```python
from build123d import *
from OCP.BRepFilletAPI import BRepFilletAPI_MakeChamfer

# Parameters (mm, degrees)
EXTRUDE_1_DEPTH     = 25
SKETCH_2_W          = 25
SKETCH_2_H          = 113.275398007
CUT_EXTRUDE_1_DEPTH = 10
EXTRUDE_1_2_DEPTH   = 25
FILLET_1_R          = 50
FILLET_2_R          = 5
CHAMFER_1_SIZE      = 3
CHAMFER_1_SIZE2     = 5.018091596
CHAMFER_1_SIZE2_2   = 4.946391741
EXTRUDE_2_DEPTH     = 25
FILLET_3_R          = 10
CHAMFER_2_SIZE      = 5


with BuildPart() as part:
    # 草图1 → Extrude 1 (new body)
    with BuildSketch(Plane.XY):
        Polygon((-40.289701428, 251), (6, 121.036629463), (6, -6), (-106, -6), (-106, 121.057565217), (-58.723691593, 251), align=None)
        Polygon((-44.521873006, 245), (0, 120), (0, 0), (-100, 0), (-100, 120), (-54.521873006, 245), align=None, mode=Mode.SUBTRACT)
    extrude(amount=EXTRUDE_1_DEPTH)

    # 草图2 → 切除-拉伸1 (cut)
    with BuildSketch(Plane(origin=(-132.504349732, 48.208397155, 0), x_dir=(0, 0, 1), z_dir=(-0.9397364726914574, 0.34189963716479416, 0))):
        with Locations((12.5, 134.158546794)):
            Rectangle(SKETCH_2_W, SKETCH_2_H)
    extrude(amount=-CUT_EXTRUDE_1_DEPTH, mode=Mode.SUBTRACT)

    # 草图4 → Extrude 1 2 (add)
    with BuildSketch(Plane.XY.offset(25)):
        Polygon((-58.077318346, 235.22759518), (-41.041186875, 235.22759518), (-39.260311955, 230.22759518), (-59.896443426, 230.22759518), align=None)
    extrude(amount=-EXTRUDE_1_2_DEPTH)

    # 圆角1
    fillet_1_edges = [part.edges().sort_by_distance(p)[0] for p in [
        (6, 121.036629463, 12.5),
    ]]
    fillet(fillet_1_edges, radius=FILLET_1_R)

    # 圆角2
    fillet_2_edges = [part.edges().sort_by_distance(p)[0] for p in [
        (-58.723691593, 251, 12.5),
        (-40.289701428, 251, 12.5),
    ]]
    fillet(fillet_2_edges, radius=FILLET_2_R)

    # 倒角1: one chamfer whose edges measure the first distance from different faces: ONE call of the kernel's chamfer builder (chamfer() names one face for all edges)
    chamfer_1_edges_1 = [part.edges().sort_by_distance(p)[0] for p in [
        (-59.896443426, 230.22759518, 12.5),
    ]]
    chamfer_1_side_1 = [part.faces().sort_by_distance(p)[0] for p in [
        (-49.57837769, 230.22759518, 12.5),
    ]]
    chamfer_1_edges_2 = [part.edges().sort_by_distance(p)[0] for p in [
        (-39.260311955, 230.22759518, 12.5),
    ]]
    chamfer_1_side_2 = [part.faces().sort_by_distance(p)[0] for p in [
        (-19.630155978, 175.11379759, 12.5),
    ]]
    chamfer_1 = BRepFilletAPI_MakeChamfer(part.part.solid().wrapped)
    for e in chamfer_1_edges_1:
        chamfer_1.Add(CHAMFER_1_SIZE, CHAMFER_1_SIZE2, e.wrapped, chamfer_1_side_1[0].wrapped)  # the first distance lies on this face
    for e in chamfer_1_edges_2:
        chamfer_1.Add(CHAMFER_1_SIZE, CHAMFER_1_SIZE2_2, e.wrapped, chamfer_1_side_2[0].wrapped)  # the first distance lies on this face
    add(Compound.cast(chamfer_1.Shape()), mode=Mode.REPLACE)

    # 草图5 → 凸台-拉伸2 (add)
    with BuildSketch(Plane.XY.offset(25)):
        Polygon((-106, 121.057565217), (-94.163375331, 130.992259513), (-90.60862045, 126.756970729), (-100, 118.874615121), align=None)
    extrude(amount=-EXTRUDE_2_DEPTH)

    # 圆角3
    fillet_3_edges = [part.edges().sort_by_distance(p)[0] for p in [
        (-106, 121.057565217, 12.5),
    ]]
    fillet(fillet_3_edges, radius=FILLET_3_R)

    # 倒角2
    chamfer_2_edges = [part.edges().sort_by_distance(p)[0] for p in [
        (0, 0, 12.5),
        (-100, 0, 12.5),
    ]]
    chamfer(chamfer_2_edges, length=CHAMFER_2_SIZE)


solid = part.part
```
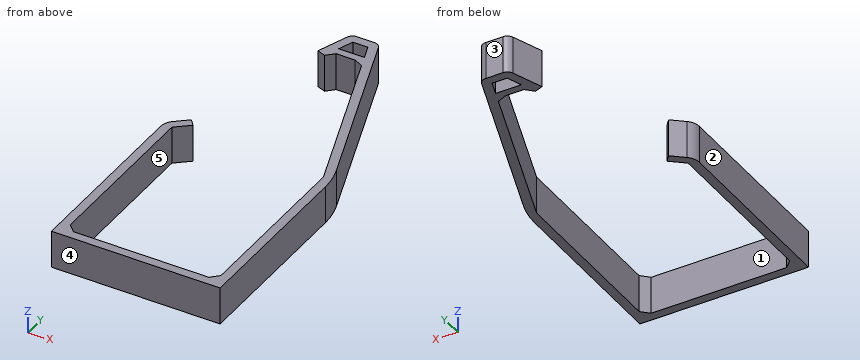
Model file for the job. Use its own axes, mm. Face numbers are marked on the shaded views. A direction names the side the tool comes from. Coordinates: 2 decimals unless noted, no trailing zeros. Write each loop counter-clockwise with the first axis right and the second up, starting at its lowest first coordinate (ties: lowest second). Pieces come first, ordered by that corner, then holes. Notation, with made-up numbers: (81, -38.75) - (109, -38.75) arc R14 ccw to (109, -19.75) - close; hole circle Ø5 at (47.5, 85.25). An arc over 180 degrees is marked (long way). Use a Markdown table: item, result. Add a question column.
Item 1: Two-plate mould, pull along Y, no slides. Class the marked faces 3, 4 and 5: pulls with the +Y half, pulls with the -Y half, needs draft (parallel to the pull), parting line crosses it, or undercut.
Item 2: Band-saw the part on A-A, the plane x = -51. Write the cut outline in (y, z), and give its area (3 significant figures).
Item 3: Band-saw the part on C-C, the plane x = -64.5. Write the cut outline in (y, z), and give its area (3 significant figures).
Item 4: 3-axis set-ups, long thin cutter, end or side, ignore diameter. For the marked faces 1 and 2: which of +Z, -Z, +X, -X, +Y, -Y reach the whole face in a straight line?
Item 5: Drop flat-ended pins along their axis: pin 1 (7.5 mm diameter, centred on x = -63, z = 17, fed in from +Y); pin 2 (8 mm diameter, centred on y = 213.5, z = 20, fed in from +X); pin 3 (5 mm diameter, centred on y = 205, z = 19, fed in from +X). Give the stop position or say it passes through.
Item 6: Band-saw the part on D-D, the plane z = 11.5. Write the cut outline in (x, y).
Item 7: Drill centre lines: line 1 along Y through (x, z) = (-50, 8.75); line 2 along X through (y, z) = (92.5, 3.5); line 3 along Y through (x, z) = (-85, 13.25). Where is each one in solid material? Low to high.
Item 8: Band-saw the part on B-B, the plane y = 95. Write the cut outline in (x, z), and give its area (3 significant figures).
A:
| question | item | result |
|---|---|---|
| 1 | face 3 | pulls with the +Y half |
| 1 | face 4 | pulls with the -Y half |
| 1 | face 5 | undercut |
| 2 | outline | (-6, 0) - (0, 0) - (0, 25) - (-6, 25) - close; (230.23, 0) - (235.23, 0) - (235.23, 25) - (230.23, 25) - close; (245, 0) - (251, 0) - (251, 25) - (245, 25) - close |
| 2 | area | 425 mm² |
| 3 | outline | (-6, 0) - (0, 0) - (0, 25) - (-6, 25) - close; (226.5, 0) - (235.12, 0) - (235.12, 25) - (226.5, 25) - close |
| 3 | area | 366 mm² |
| 4 | face 1 | +Z, -Z |
| 4 | face 2 | +Z, -Z, -X, +Y, -Y |
| 5 | pin 1 | stops at y = 248.96 |
| 5 | pin 2 | stops at x = -25.51 |
| 5 | pin 3 | stops at x = -23.02 |
| 6 | outline | (-106, -6) - (6, -6) - (6, 112.4) arc R50 ccw to (3.1, 129.17) - (-39.11, 247.68) arc R5 ccw to (-43.82, 251) - (-55.22, 251) arc R5 ccw to (-59.92, 247.71) - (-67.27, 227.51) - (-61.63, 225.46) - (-61.61, 225.51) - (-56.9, 230.23) - (-44.21, 230.23) - (-38.25, 227.4) - (0, 120) - (0, 5) - (-5, 0) - (-95, 0) - (-100, 5) - (-100, 118.87) - (-90.61, 126.76) - (-94.16, 130.99) - (-102.43, 124.05) arc R10 ccw to (-106, 116.4) - close; hole (-58.08, 235.23) - (-41.04, 235.23) - (-44.52, 245) - (-54.52, 245) - close |
| 7 | line 1 | y = -6 to 0, 230.23 to 235.23, 245 to 251 |
| 7 | line 2 | x = -106 to -100, 0 to 6 |
| 7 | line 3 | y = -6 to 0 |
| 8 | outline | (-106, 0) - (-100, 0) - (-100, 25) - (-106, 25) - close; (0, 0) - (6, 0) - (6, 25) - (0, 25) - close |
| 8 | area | 300 mm² |
